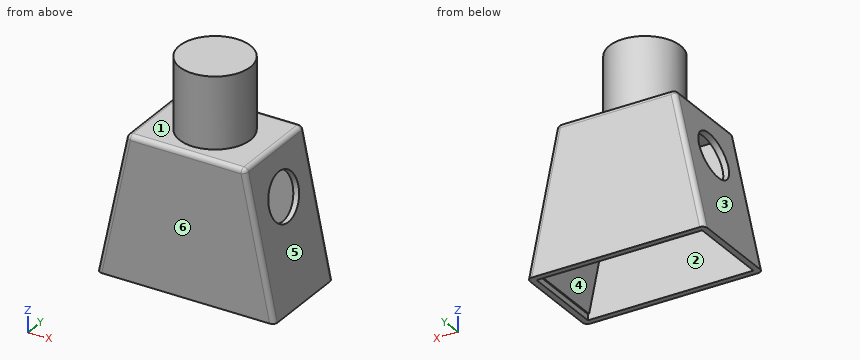
```python
from build123d import *

# Parameters (mm, degrees)
F1_DEPTH = 8
F2_T     = -0.5
F3_W     = 13.9785291107
F3_H     = 7
F4_DEPTH = 0.5
F5_R     = 0.4
F6_R     = 2
F7_DEPTH = 1
F8_R     = 3
F9_DEPTH = 6


# Not quite as in the source:
# - a pattern or mirror of a feature is missing from the dataset's text; its kind, count and spacing are read off the source's solid


with BuildPart() as f1:
    # F0 (on Front) → F1 (new body)
    with BuildSketch(Plane.XZ):
        Polygon((-7.5, 0), (0, 0), (7.5, 0), (5, 12), (0, 12), (-5, 12), align=None)
    extrude(amount=F1_DEPTH)

    # F2
    f2_openings = [f1.faces().sort_by_distance(p)[0] for p in [
        (0, -4, 0),
    ]]
    offset(amount=F2_T, openings=f2_openings)

    # F3 (on face) → F4 (cut)
    with BuildSketch(Plane(origin=(0, 0, 0), x_dir=(1, 0, 0), z_dir=(0, 0, -1))):
        with Locations((0, 4)):
            Rectangle(F3_W, F3_H)
    extrude(amount=-F4_DEPTH, mode=Mode.SUBTRACT)

    # F5
    f5_edges = [f1.edges().sort_by_distance(p)[0] for p in [
        (6.25, -8, 6),
        (5, -4, 12),
        (0, -8, 12),
        (6.25, 0, 6),
        (0, 0, 12),
        (-6.25, 0, 6),
        (-5, -4, 12),
        (-6.25, -8, 6),
    ]]
    fillet(f5_edges, radius=F5_R)

    # F6 (on face) → F7 (cut)
    with BuildSketch(Plane(origin=(-7.1880199667, 0, 1.4975041597), x_dir=(0, -1, 0), z_dir=(-0.9789804197, 0, 0.2039542541))):
        with Locations((4, 6.8027387439)):
            Circle(F6_R)
    f7 = extrude(amount=-F7_DEPTH, mode=Mode.SUBTRACT)

    # F7_copies: F7 across plane
    add(f7.mirror(Plane(origin=(0, 0, 0), x_dir=(0, 0, 1), z_dir=(1, 0, 0))), mode=Mode.SUBTRACT)

    # F8 (on face) → F9 (join)
    with BuildSketch(Plane.XY.offset(12)):
        with Locations((0, -4)):
            Circle(F8_R)
    extrude(amount=F9_DEPTH)


solid = f1.part
```
Design review of the part built by this model. Coordinates are the model's own, in mm. Face numbers are marked on the shaded views. A direction names the side the tool comes from. Round coordinates to 2 decimals unless told otherwise and drop trailing zeros. Write each loop counter-clockwise with the first axis right and the second up, starting at its lowest first coordinate (ties: lowest second). Pieces come first, ordered by that corner, then holes. Notation, with made-up numbers: (20.25, -26.75) -> (55.25, -26.75) arc R20 cw to (55.25, -5.75) -> close; hole circle Ø11 at (-35, -11). An arc over 180 degrees is marked (long way). Write item = value, one per line. Start each with the question number.
1) Wall thickness on probe 1 along Y at (x, z) = (2.5, 1.25); probe 2 along Z at (x, y) = (3, -3); probe 3 along X at (y, z) = (-1.25, 2.5): over which ranges is each line inside the solid? List them lowest first. Write a range as from..to.
2) Tool access review of the marked faces 1, 2 and 3: name each direction out of +Z, -Z, +X, -X, +Y, -Y from which nothing blocks a thin tool from reaching the whole face with its end or side.
3) Take a section at A-A, the plane x = 0. State the section outline as (y, z) points.
4) Take a section at C-C, the plane y = -2.25. State the section outline as (x, z) points, plus the area to 3 significant figures.
5) Mouldability with a two-part tool opening along Y and no side actions: class the marked faces 4, 5 and 6 as +Y half, -Y half, draft (parallel to the pull), parting line (faces both ways), or undercut.
6) Clearance check with flat-ended pins moving along their axes: pin 1 (2 mm diameter, centred on y = -6.5, z = 2, fed in from -X); pin 2 (4 mm diameter, centred on x = 5, y = -7, fed in from +Z); pin 3 (4 mm diameter, centred on y = -2, z = 11.5, fed in from +X). State where each tip first meets the part, or that it passes through.
7) Take a section at B-B, the plane y = -4. State the section outline as (x, z) points.
Results list:
q1.probe_1 = -8..-7.5, -0.5..0
q1.probe_2 = 11.5..12
q1.probe_3 = -6.98..-6.47, 6.47..6.98
q2.face_1 = +Z
q2.face_2 = -Z
q2.face_3 = +Z, -X, +Y, -Y
q3.outline = (-8, 0) -> (-7.5, 0) -> (-7.5, 11.5) -> (-0.5, 11.5) -> (-0.5, 0) -> (0, 0) -> (0, 11.6) arc R0.4 ccw to (-0.4, 12) -> (-1, 12) -> (-1, 18) -> (-7, 18) -> (-7, 12) -> (-7.6, 12) arc R0.4 ccw to (-8, 11.6) -> close
q4.outline = (-7.5, 0) -> (-6.99, 0) -> (-6.99, 0.5) -> (-6.89, 0.5) -> (-5.51, 7.11) -> (-6, 7.21) -> close; (-5.6, 9.11) -> (-5.11, 9) -> (-4.59, 11.5) -> (4.59, 11.5) -> (5.11, 9) -> (5.6, 9.11) -> (5.07, 11.68) arc R0.4 ccw to (4.67, 12) -> (2.44, 12) -> (2.44, 18) -> (-2.44, 18) -> (-2.44, 12) -> (-4.67, 12) arc R0.4 ccw to (-5.07, 11.68) -> close; (5.51, 7.11) -> (6.89, 0.5) -> (6.99, 0.5) -> (6.99, 0) -> (7.5, 0) -> (6, 7.21) -> close
q4.area = 44.0 mm²
q5.face_4 = undercut
q5.face_5 = draft
q5.face_6 = -Y half
q6.pin_1 = -7.29
q6.pin_2 = 12
q6.pin_3 = 5.52
q7.outline = (-7.5, 0) -> (-6.99, 0) -> (-6.99, 0.5) -> (-6.89, 0.5) -> (-5.72, 6.1) -> (-6.21, 6.2) -> close; (-5.39, 10.12) -> (-4.9, 10.01) -> (-4.59, 11.5) -> (4.59, 11.5) -> (4.9, 10.01) -> (5.39, 10.12) -> (5.07, 11.68) arc R0.4 ccw to (4.67, 12) -> (3, 12) -> (3, 18) -> (-3, 18) -> (-3, 12) -> (-4.67, 12) arc R0.4 ccw to (-5.07, 11.68) -> close; (5.72, 6.1) -> (6.89, 0.5) -> (6.99, 0.5) -> (6.99, 0) -> (7.5, 0) -> (6.21, 6.2) -> close
